Check sheet for the modelled part. Datum: model origin and axes. Units: mm. Round coordinates to 2 decimals unless told otherwise and drop trailing zeros.
Autodesk Fusion 360 part; units mm, degrees
sketch "Sketch1" plane through (0, 0, 0) normal (0, 0, 1) x (1, 0, 0)
  line L0 (-102.5159, 0.7104) -> (97.4841, 0.7104) construction
  line L1 (0, 100) -> (0, -100) construction
  line L2 (-60, 65.7104) -> (60, 65.7104)
  line L3 (60, 65.7104) -> (60, -64.2896)
  line L4 (60, -64.2896) -> (-60, -64.2896)
  line L5 (-60, -64.2896) -> (-60, 65.7104)
  line L6 (60, 30.7104) -> (39.4499, 30.7104) construction
  line L7 (39.4499, 30.7104) -> (39.4499, -29.2896) construction
  line L8 (39.4499, -29.2896) -> (60, -29.2896) construction
  line L9 (60, -29.2896) -> (60, 30.7104) construction
  line L10 (49.7249, 30.7104) -> (49.7249, -29.2896) construction
  line L11 (56.4749, 30.7104) -> (42.9749, 30.7104) construction
  line L12 (42.9749, 30.7104) -> (42.9749, -29.2896) construction
  line L13 (42.9749, -29.2896) -> (56.4749, -29.2896) construction
  line L14 (56.4749, -29.2896) -> (56.4749, 30.7104) construction
  line L15 (-56.4749, -29.2896) -> (-56.4749, 30.7104) construction
  line L16 (-42.9749, 30.7104) -> (-42.9749, -29.2896) construction
  line L17 (-60, 30.7104) -> (-39.4499, 30.7104) construction
  line L18 (-42.9749, -29.2896) -> (-56.4749, -29.2896) construction
  line L19 (-39.4499, 30.7104) -> (-39.4499, -29.2896) construction
  line L20 (-49.7249, 30.7104) -> (-49.7249, -29.2896) construction
  line L21 (-39.4499, -29.2896) -> (-60, -29.2896) construction
  line L22 (39.4499, 43.2104) -> (-16.5501, 43.2104) construction
  line L23 (-16.5501, 43.2104) -> (-16.5501, -41.7896) construction
  line L24 (-16.5501, -41.7896) -> (39.4499, -41.7896) construction
  line L25 (39.4499, -41.7896) -> (39.4499, 43.2104) construction
  line L26 (35.9499, 40) -> (-13.0501, 40) construction
  line L27 (-13.0501, 40) -> (-13.0501, -18) construction
  line L28 (-13.0501, -18) -> (35.9499, -18) construction
  line L29 (35.9499, -18) -> (35.9499, 40) construction
  line L30 (11.4499, 43.2104) -> (11.4499, -41.7896) construction
  dimension "d1" = 200
  dimension "d2" = 200
  dimension "d3" = 120
  dimension "d4" = 130
  dimension "d5" = 60
  dimension "d6" = 13.5
  dimension "d7" = 56
  dimension "d8" = 85
  dimension "d9" = 49
  dimension "d10" = 58
extrude "Extrude1" add sketch "Sketch1" along normal blind 5
hole "Hole1" at (56.4749, 30.7104, 0) at (42.9749, 30.7104, 0) at (42.9749, -29.2896, 0) at (56.4749, -29.2896, 0) at (-42.9749, 30.7104, 0) at (-56.4749, 30.7104, 0) at (-56.4749, -29.2896, 0) at (-42.9749, -29.2896, 0) direction (0, 0, 1) diameter 3 depth 5 tip angle 180
hole "Hole2" at (35.9499, 40, 0) at (35.9499, -18, 0) at (-13.0501, 40, 0) at (-13.0501, -18, 0) direction (0, 0, 1) diameter 2.5 depth 5 tip angle 180
Item 1: Release check for a two-part mould opening along X. For faces 1 (the cylindrical face through (-43.04, 29.21, 2.54)), 2 (the flat face through (-1, 2, 5)), 3 (the flat face through (-60, 0, 2)) record: released by +X, released by -X, zero draft, split by the parting line, or undercut.
Answer:
face 1: undercut
face 2: zero draft
face 3: released by -X
Item 2: Go/stop test with flat-tipped pins: P1, Ø4, axis at x = 35.95, y = 40, coming from the -Z side; P2, Ø1.5, axis at x = 35.95, y = -18, coming from the -Z side. Record where each tip stops, or that it passes through.
Answer:
P1: stops at z = 0
P2: passes through
Item 3: Scan lines: line 1 along X through (y, z) = (40, 3.3); line 2 along X through (y, z) = (31, 1.75); line 3 along X through (y, z) = (29.5, 3.5). Record each from-to range of solid material in increasing order.
Answer:
line 1: x = -60 to -14.3, -11.8 to 34.7, 37.2 to 60
line 2: x = -60 to -57.95, -55 to -44.45, -41.5 to 41.5, 44.45 to 55, 57.95 to 60
line 3: x = -60 to -57.36, -55.59 to -43.86, -42.09 to 42.09, 43.86 to 55.59, 57.36 to 60
